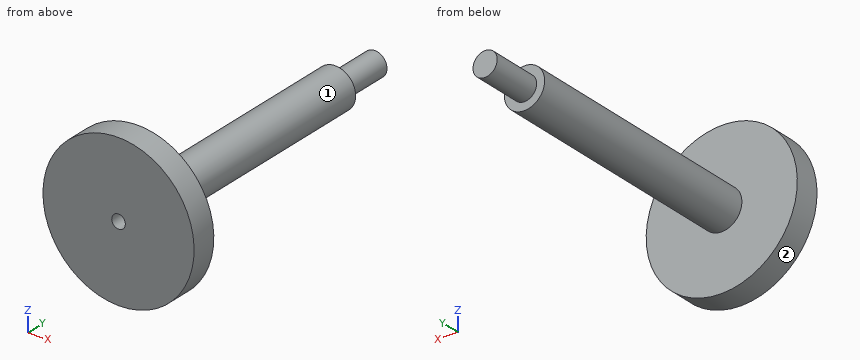
```python
from build123d import *

# Parameters (mm, degrees)
CROQUIS2_R            = 1.35
CORTAR_EXTRUIR1_DEPTH = 20


with BuildPart() as part:
    # Croquis1 → Revolución1 (revolve)
    with BuildSketch(Plane(origin=(0, 0, 0), x_dir=(0, 0, -1), z_dir=(1, 0, 0)), mode=Mode.PRIVATE) as revoluci_n1_sk:
        Polygon((0, 0), (-2.4, 0), (-2.4, -10), (-4, -10), (-4, -60), (-15, -60), (-15, -65), (0, -65), align=None)
    revolve(revoluci_n1_sk.sketch.rotate(Axis((0, -65, 0), (0, 1, 0)), 180), axis=Axis((0, -65, 0), (0, 1, 0)))

    # Croquis2 → Cortar-Extruir1 (cut)
    with BuildSketch(Plane.XZ.offset(65)):
        with Locations(Location((0, 0, 0), (0, 0, 270))):
            Circle(CROQUIS2_R)
    extrude(amount=-CORTAR_EXTRUIR1_DEPTH, mode=Mode.SUBTRACT)


solid = part.part
```
Check sheet for the modelled part. Datum: model origin and axes. Units: mm. Face numbers are marked on the shaded views. A direction names the side the tool comes from. Round coordinates to 2 decimals unless told otherwise and drop trailing zeros. Order: outer loops, then holes, each group sorted by start corner. A loop starts at its lowest first (then second) coordinate and runs counter-clockwise, first axis right, second up.
1) Section check B-B (z = 0). Record the boundary of the cut face in (x, y).
2) Tool access check on the marked faces 1 and 2. Record the directions out of +Z, -Z, +X, -X, +Y, -Y that give a thin tool (end or side, any length) a straight path to the whole face; none if there is none.
3) Scan lines: line 1 (X direction, y = -59.5, z = 0); line 2 (Y direction, x = 11.75, z = 0.25); line 3 (Z direction, x = 1.5, y = -25). Record each from-to range of solid material in increasing order.
4) Go/stop test with flat-tipped pins: pin 1 Ø10 at (y, z) = (-46, -2) entering from -X; pin 2 Ø9 at (x, z) = (-7, -2) entering from +Y; pin 3 Ø8 at (x, z) = (-11, -10.5) entering from +Y. Record where each tip stops, or that it passes through.
5) Section check D-D (y = -17). Record the boundary of the cut face in (x, z), and give its area (3 significant figures).
6) Section check C-C (x = 0). Record the boundary of the cut face in (y, z), and give its area (3 significant figures).
7) Section check A-A (y = -53). Record the boundary of the cut face in (x, z), and give its area (3 significant figures).
Result:
1. outline: (-15, -65) - (-1.35, -65) - (-1.35, -45) - (1.35, -45) - (1.35, -65) - (15, -65) - (15, -60) - (4, -60) - (4, -10) - (2.4, -10) - (2.4, 0) - (-2.4, 0) - (-2.4, -10) - (-4, -10) - (-4, -60) - (-15, -60) - close
2. face 1: +Y
2. face 2: +Y, -Y
3. line 1: x = -4 to -1.35, 1.35 to 4
3. line 2: y = -65 to -60
3. line 3: z = -3.71 to 3.71
4. pin 1: stops at x = -4
4. pin 2: stops at y = -10
4. pin 3: stops at y = -60
5. outline: circle Ø8 at (0, 0)
5. area: 50.3 mm2
6. outline: (-65, -15) - (-60, -15) - (-60, -4) - (-10, -4) - (-10, -2.4) - (0, -2.4) - (0, 2.4) - (-10, 2.4) - (-10, 4) - (-60, 4) - (-60, 15) - (-65, 15) - (-65, 1.35) - (-45, 1.35) - (-45, -1.35) - (-65, -1.35) - close
6. area: 544 mm2
7. outline: circle Ø8 at (0, 0); hole circle Ø2.7 at (0, 0)
7. area: 44.5 mm2
